Geometry check sheet. Reference: the model listing, model coordinates, mm. A direction names the side the tool comes from. Give positions to 0.01 mm unless a question says otherwise; leave off trailing zeros. Loops run counter-clockwise (first coordinate to the right, second up) from the corner with the lowest first, then second, coordinate; pieces in that order, holes last. Notation, with made-up numbers: (51, -16.75) - (104, -16.75) arc R22 ccw to (104, 0.25) - close; hole circle Ø2 at (-11.5, 62). An arc over 180 degrees is marked (long way). Use a Markdown table: item, result. Add a question column.
1. Draft check along X on faces 3 (the flat face through (-10.901, -9, 56)), 4 (the cylindrical face through (0.3, -34.15, 61.79)), 5 (the flat face through (0, 16.007, 56)), 6 (the flat face through (-12.171, -10, 56)). Enter one of: pulls with the +X half, pulls with the -X half, needs draft (parallel to the pull), parting line crosses it, or undercut.
2. Cross-section at A-A on z = 88.9. Enter the section's corners in (x, y).
3. Cross-section at C-C on y = -16. Enter the section's corners in (x, z), and give its area (3 significant figures).
4. Material ranges on L1, parallel to Y at x = 3.75, z = 72; L2, parallel to X at y = -2.5, z = 35.5; L3, parallel to X at y = 15.3, z = 88.9, recorded low to high.
5. Set-up check for faces 1 (the flat face through (11.959, -10, 56)), 2 (the cylindrical face through (0.3, -34.15, 10.99)): record each of +Z, -Z, +X, -X, +Y, -Y from which the full face is reachable in a straight line by a thin tool's end or side.
6. Depth check by flat-ended pin: P1, Ø2, axis at x = 0.53, z = 63.5, coming from the +Y side (1 decimal). Enter the tip coordinate at first touch or a pass-through.
7. Cross-section at B-B on x = -9. Enter the section's corners in (y, z).
Autodesk Inventor part; units mm, degrees
ref_plane "YZ Plane" through (0, 0, 0) normal (1, 0, 0) x (0, 1, 0)
ref_plane "XZ Plane" through (0, 0, 0) normal (0, 1, 0) x (-1, 0, 0)
ref_plane "XY Plane" through (0, 0, 0) normal (0, 0, 1) x (1, 0, 0)
sketch "Sketch1" plane through (0, 0, 0) normal (0, 0, 1) x (1, 0, 0)
  line L0 (-12.1708, 16.0073) -> (13.2292, 16.0073)
  line L1 (13.2292, 16.0073) -> (13.2292, -34.7927)
  line L2 (13.2292, -34.7927) -> (-12.1708, -34.7927)
  line L3 (-12.1708, -34.7927) -> (-12.1708, 16.0073)
  line L4 (11.9592, 14.7373) -> (-10.9008, 14.7373)
  line L5 (-10.9008, 14.7373) -> (-10.9008, -33.5227)
  line L6 (-10.9008, -33.5227) -> (11.9592, -33.5227)
  line L7 (11.9592, -33.5227) -> (11.9592, 14.7373)
  point P0 (0, 0)
  dimension "d0" = 25.4
  dimension "d1" = 50.8
  dimension "d2" = 1.27
extrude "Extrusion1" add sketch "Sketch1" along normal blind 114.3
sketch "Sketch2" plane through (-12.1708, 16.0073, 0) normal (0, 1, 0) x (1, 0, 0)
  circle A0 centre (12.7, -12.7) radius 1.7272
  line L0 (25.4, 0) -> (0, 0)
  line L1 (0, 0) -> (0, -114.3)
  point P0 (12.1708, 0)
  dimension "d5" = 3.4544
  dimension "d6" = 12.7
  dimension "d7" = 12.7
extrude "Extrusion2" cut sketch "Sketch2" against normal through all
pattern_linear "Rectangular Pattern1" count 11 spacing 25.4 along (0, 0, 1) of "Extrusion2"
equation "\"d3\" = d13"
equation "\"d10\" = d14"
equation "\"d13\" = 114.3"
equation "\"d14\" = d13"
properties part number "VersaFrame (Gripper-MovingLong)"
Values found:
| question | item | result |
|---|---|---|
| 1 | face 3 | undercut |
| 1 | face 4 | undercut |
| 1 | face 5 | needs draft |
| 1 | face 6 | pulls with the -X half |
| 2 | outline | (-12.17, -34.79) - (-1.2, -34.79) - (-1.2, -33.52) - (-10.9, -33.52) - (-10.9, 14.74) - (-1.2, 14.74) - (-1.2, 16.01) - (-12.17, 16.01) - close; (2.26, -34.79) - (13.23, -34.79) - (13.23, 16.01) - (2.26, 16.01) - (2.26, 14.74) - (11.96, 14.74) - (11.96, -33.52) - (2.26, -33.52) - close |
| 3 | outline | (-12.17, 0) - (-10.9, 0) - (-10.9, 114.3) - (-12.17, 114.3) - close; (11.96, 0) - (13.23, 0) - (13.23, 114.3) - (11.96, 114.3) - close |
| 3 | area | 290 mm2 |
| 4 | L1 | y = -34.79 to -33.52, 14.74 to 16.01 |
| 4 | L2 | x = -12.17 to -10.9, 11.96 to 13.23 |
| 4 | L3 | x = -12.17 to -1.2, 2.26 to 13.23 |
| 5 | face 1 | +Z, -Z |
| 5 | face 2 | +Y, -Y |
| 6 | P1 | passes through |
| 7 | outline | (-34.79, 0) - (-33.52, 0) - (-33.52, 114.3) - (-34.79, 114.3) - close; (14.74, 0) - (16.01, 0) - (16.01, 114.3) - (14.74, 114.3) - close |
